```python
from build123d import *

# Parameters (mm, degrees)
F0_R         = 2.5
F1_DEPTH     = 15
F0_W         = 15
F0_H         = 28
F2_DEPTH     = 40
F3_DEPTH     = 30
F4_T1_DEPTH  = 15
F4_T3_DEPTH  = 40
F4_T5_DEPTH  = 80
F4_T8_ANGLE  = 90
F4_T10_ANGLE = 90
F4_T12_ANGLE = 90
F4_T14_ANGLE = 90
F5_R         = 7


# Not quite as in the source:
# - a fillet or chamfer that OpenCascade refuses, or shapes differently, is made with other operations: its cross-section is extruded or revolved along the edge and cut away or added


with BuildPart() as f1:
    # F0 (on Top) → F1 (new body)
    with BuildSketch(Plane.XY):
        with BuildLine():
            ThreePointArc((-25, -40), (-23.5355339059, -43.5355339059), (-20, -45))
            Line((-20, -45), (20, -45))
            ThreePointArc((20, -45), (23.5355339059, -43.5355339059), (25, -40))
            Line((25, -40), (25, 40))
            ThreePointArc((25, 40), (23.5355339059, 43.5355339059), (20, 45))
            Line((20, 45), (-20, 45))
            ThreePointArc((-20, 45), (-23.5355339059, 43.5355339059), (-25, 40))
            Line((-25, 40), (-25, -40))
        make_face()
        with Locations((-20, -40)):
            Circle(F0_R, mode=Mode.SUBTRACT)
        with Locations((20, -40)):
            Circle(F0_R, mode=Mode.SUBTRACT)
        with Locations((-20, 40)):
            Circle(F0_R, mode=Mode.SUBTRACT)
        Polygon((7.5, 28), (7.5, 0), (7.5, -28), (-7.5, -28), (-7.5, 0), (-7.5, 28), align=None, mode=Mode.SUBTRACT)
        with Locations((20, 40)):
            Circle(F0_R, mode=Mode.SUBTRACT)
    extrude(amount=F1_DEPTH)

    # F0 (on Top) → F2 (join)
    with BuildSketch(Plane.XY):
        with Locations((0, 14)):
            Rectangle(F0_W, F0_H)
    extrude(amount=F2_DEPTH)

    # F0 (on Top) → F3 (join)
    with BuildSketch(Plane.XY):
        with Locations((0, -14)):
            Rectangle(F0_W, F0_H)
    extrude(amount=F3_DEPTH)

    # F4: fillet of radius 5 on 6 edges, made by hand

    # F4_s2 → F4_t1 (join)
    with BuildSketch(Plane.YZ.offset(-7.5)):
        with BuildLine():
            ThreePointArc((0, 35), (-1.4644660941, 31.4644660941), (-5, 30))
            Line((-5, 30), (0, 30))
            Line((0, 30), (0, 35))
        make_face()
    extrude(amount=F4_T1_DEPTH)

    # F4_s4 → F4_t3 (cut)
    with BuildSketch(Plane.YZ.offset(-20)):
        with BuildLine():
            ThreePointArc((0, 35), (1.4644660941, 38.5355339059), (5, 40))
            Line((5, 40), (0, 40))
            Line((0, 40), (0, 35))
        make_face()
        with BuildLine():
            ThreePointArc((28, 35), (26.5355339059, 38.5355339059), (23, 40))
            Line((23, 40), (28, 40))
            Line((28, 40), (28, 35))
        make_face()
        with BuildLine():
            ThreePointArc((-45, 10), (-43.5355339059, 13.5355339059), (-40, 15))
            Line((-40, 15), (-45, 15))
            Line((-45, 15), (-45, 10))
        make_face()
        with BuildLine():
            ThreePointArc((-28, 25), (-26.5355339059, 28.5355339059), (-23, 30))
            Line((-23, 30), (-28, 30))
            Line((-28, 30), (-28, 25))
        make_face()
        with BuildLine():
            ThreePointArc((40, 15), (43.5355339059, 13.5355339059), (45, 10))
            Line((45, 10), (45, 15))
            Line((45, 15), (40, 15))
        make_face()
    extrude(amount=F4_T3_DEPTH, mode=Mode.SUBTRACT)

    # F4_s6 → F4_t5 (cut)
    with BuildSketch(Plane.XZ.offset(-40)):
        with BuildLine():
            ThreePointArc((-25, 10), (-23.5355339059, 13.5355339059), (-20, 15))
            Line((-20, 15), (-25, 15))
            Line((-25, 15), (-25, 10))
        make_face()
        with BuildLine():
            ThreePointArc((20, 15), (23.5355339059, 13.5355339059), (25, 10))
            Line((25, 10), (25, 15))
            Line((25, 15), (20, 15))
        make_face()
    extrude(amount=F4_T5_DEPTH, mode=Mode.SUBTRACT)

    # F4_s7 → F4_t8 (revolve, cut)
    with BuildSketch(Plane.XZ.offset(40)):
        with BuildLine():
            ThreePointArc((-25, 10), (-23.5355339059, 13.5355339059), (-20, 15))
            Line((-20, 15), (-25, 15))
            Line((-25, 15), (-25, 10))
        make_face()
    revolve(axis=Axis((-20, -40, 15), (0, 0, 1)), revolution_arc=F4_T8_ANGLE, mode=Mode.SUBTRACT)

    # F4_s9 → F4_t10 (revolve, cut)
    with BuildSketch(Plane.YZ.offset(-20)):
        with BuildLine():
            ThreePointArc((40, 15), (43.5355339059, 13.5355339059), (45, 10))
            Line((45, 10), (45, 15))
            Line((45, 15), (40, 15))
        make_face()
    revolve(axis=Axis((-20, 40, 15), (0, 0, 1)), revolution_arc=F4_T10_ANGLE, mode=Mode.SUBTRACT)

    # F4_s11 → F4_t12 (revolve, cut)
    with BuildSketch(Plane.XZ.offset(-40)):
        with BuildLine():
            ThreePointArc((20, 15), (23.5355339059, 13.5355339059), (25, 10))
            Line((25, 10), (25, 15))
            Line((25, 15), (20, 15))
        make_face()
    revolve(axis=Axis((20, 40, 15), (0, 0, 1)), revolution_arc=F4_T12_ANGLE, mode=Mode.SUBTRACT)

    # F4_s13 → F4_t14 (revolve, cut)
    with BuildSketch(Plane.YZ.offset(20)):
        with BuildLine():
            ThreePointArc((-40, 15), (-43.5355339059, 13.5355339059), (-45, 10))
            Line((-45, 10), (-45, 15))
            Line((-45, 15), (-40, 15))
        make_face()
    revolve(axis=Axis((20, -40, 15), (0, 0, 1)), revolution_arc=F4_T14_ANGLE, mode=Mode.SUBTRACT)

    # F5
    f5_edges = [f1.edges().sort_by_distance(p)[0] for p in [
        (-7.5, 0, 15),
        (7.5, 0, 15),
    ]]
    fillet(f5_edges, radius=F5_R)


solid = f1.part
```
CAD build for the part. Positions are in the model's coordinates, mm. A direction names the side the tool comes from. Round coordinates to 2 decimals unless told otherwise and drop trailing zeros. Loops run counter-clockwise (first coordinate to the right, second up) from the corner with the lowest first, then second, coordinate; pieces in that order, holes last. Notation, with made-up numbers: (15, -31.5) - (39, -31.5) arc R30 cw to (39, 3.5) - close; hole circle Ø4 at (26.5, 1). An arc over 180 degrees is marked (long way). Return JSON: item names as keys, results as strings. Group by question number.
Q1. Two-plate mould, pull along Y, no slides. Class faces 5 (the face through (0, 27, 38)), 6 (the face through (18, 38.5, 7.4)), 7 (the face through (25, -1, 5)), 8 (the face through (-22.5, -39.9, 7.4)): +Y half, -Y half, draft (parallel to the pull), parting line (faces both ways), or undercut.
Q2. Band-saw the part on D-D on y = -19.5. Give the cut face in (x, z), plus the area to 3 significant figures.
Q3. Flat gauge pins, fed straight in: pin 1 Ø5 at (x, z) = (-1.5, 18.5) entering from -Y; pin 2 Ø6 at (x, z) = (-4.5, 29.5) entering from +Y; pin 3 Ø1 at (y, z) = (-24.5, 28) entering from -X; pin 4 Ø3 at (x, y) = (-20, -40) entering from +Z. Where does each tip first touch, or does it go through?
Q4. Band-saw the part on A-A on z = 8.5. Give the cut face in (x, y).
Q5. Drill centre lines: line 1 along Y through (x, z) = (20, 8); line 2 along Z through (x, y) = (-17.5, -17.5); line 3 along X through (y, z) = (-22, 22). Where is each one in solid material? Low to high. Write a range as [from, to].
Q6. Band-saw the part on B-B on y = 26. Give the cut face in (x, z), plus the area to 3 significant figures.
Q7. Band-saw the part on C-C on x = 2.5. Give the cut face in (y, z).
Q8. Tool access for faces 1 (the face through (-7.5, 6, 29)), 2 (the face through (0, 28, 25)), 3 (the face through (7.5, 6, 29)), 4 (the face through (17, 1, 15)): list every direction of +Z, -Z, +X, -X, +Y, -Y with a clear straight run to the whole face (end or side of a thin tool).
Solutions:
{
 "1": {"face 5": "+Y half", "face 6": "undercut", "face 7": "draft", "face 8": "undercut"},
 "2": {"outline": "(-25, 0) - (25, 0) - (25, 10) arc R5 ccw to (20, 15) - (14.5, 15) arc R7 cw to (7.5, 22) - (7.5, 30) - (-7.5, 30) - (-7.5, 22) arc R7 cw to (-14.5, 15) - (-20, 15) arc R5 ccw to (-25, 10) - close", "area": "985 mm^2"},
 "3": {"pin 1": "stops at y = -28", "pin 2": "stops at y = 28", "pin 3": "stops at x = -7.5", "pin 4": "passes through"},
 "4": {"outline": "(-25, -40) arc R5 ccw to (-20, -45) - (20, -45) arc R5 ccw to (25, -40) - (25, 40) arc R5 ccw to (20, 45) - (-20, 45) arc R5 ccw to (-25, 40) - close; hole circle Ø5 at (-20, -40); hole circle Ø5 at (-20, 40); hole circle Ø5 at (20, -40); hole circle Ø5 at (20, 40)"},
 "5": {"line 1": "y = [-45, -42.5], [-37.5, 37.5], [42.5, 45]", "line 2": "z = [0, 15]", "line 3": "x = [-7.5, 7.5]"},
 "6": {"outline": "(-25, 0) - (25, 0) - (25, 10) arc R5 ccw to (20, 15) - (14.5, 15) arc R7 cw to (7.5, 22) - (7.5, 39) - (-7.5, 39) - (-7.5, 22) arc R7 cw to (-14.5, 15) - (-20, 15) arc R5 ccw to (-25, 10) - close", "area": "1,120 mm^2"},
 "7": {"outline": "(-45, 0) - (45, 0) - (45, 10) arc R5 ccw to (40, 15) - (28, 15) - (28, 35) arc R5 ccw to (23, 40) - (5, 40) arc R5 ccw to (0, 35) arc R5 cw to (-5, 30) - (-23, 30) arc R5 ccw to (-28, 25) - (-28, 15) - (-40, 15) arc R5 ccw to (-45, 10) - close"},
 "8": {"face 1": "+Z, -X, +Y, -Y", "face 2": "+Z, +X, -X, +Y", "face 3": "+Z, +X, +Y, -Y", "face 4": "+Z"}
}
